Build history of the part. All positions in model axes, mm. Face numbers are marked on the shaded views. A direction names the side the tool comes from. Round coordinates to 2 decimals unless told otherwise and drop trailing zeros. Order: outer loops, then holes, each group sorted by start corner. A loop starts at its lowest first (then second) coordinate and runs counter-clockwise, first axis right, second up. Notation, with made-up numbers: (78.25, 48) -> (110.25, 48) arc R23 ccw to (110.25, 83) -> close; hole circle Ø8 at (-17, -25). An arc over 180 degrees is marked (long way). Write item = value, one per line.
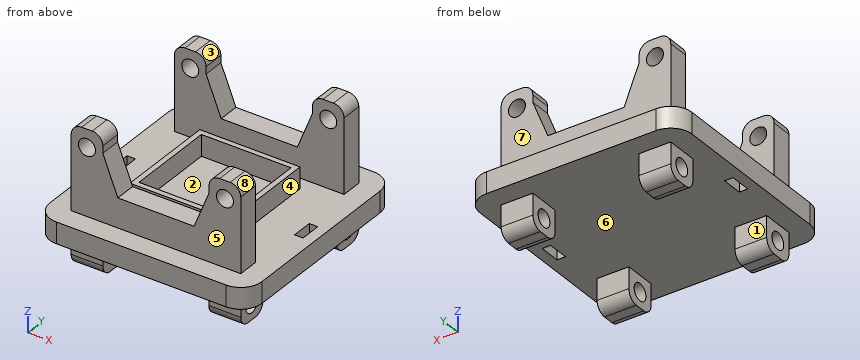
from build123d import *

# Parameters (mm, degrees)
SCHIZZO1_W                   = 100
SCHIZZO1_H                   = 100
ESTRUSIONE_ESTRUSIONE1_DEPTH = 10
RACCORDO1_R                  = 10
SCHIZZO6_W                   = 15
SCHIZZO6_H                   = 15
ESTRUSIONE_ESTRUSIONE2_DEPTH = 15
RACCORDO2_R                  = 5
SCHIZZO7_R                   = 4
TAGLIO_ESTRUSIONE1_DEPTH     = 15
RACCORDO3_R                  = 5
SPECCHIA6_COPY_1_SKETCH_W    = 15
SPECCHIA6_COPY_1_SKETCH_H    = 15
SPECCHIA6_COPY_1_DEPTH       = 15
SPECCHIA6_COPY_2_SKETCH_R    = 4
SPECCHIA6_COPY_2_DEPTH       = 15
RACCORDO3_OF_SPECCHIA6_R     = 5
RACCORDO4_R                  = 5
SCHIZZO8_W                   = 47.3
SCHIZZO8_H                   = 47.3
SCHIZZO8_W_2                 = 42.3
SCHIZZO8_H_2                 = 42.3
ESTRUSIONE_ESTRUSIONE4_DEPTH = 10
SCHIZZO10_W                  = 80
SCHIZZO10_H                  = 10
ESTRUSIONE_ESTRUSIONE6_DEPTH = 40
SCHIZZO11_R                  = 4
TAGLIO_ESTRUSIONE4_DEPTH     = 30
SCHIZZO11_4_R                = 4
TAGLIO_ESTRUSIONE5_DEPTH     = 30
RACCORDO5_R                  = 5
RACCORDO6_R                  = 5
TAGLIO_ESTRUSIONE6_DEPTH     = 30
RACCORDO7_R                  = 5
RACCORDO8_R                  = 5
RACCORDO9_R                  = 5
SCHIZZO15_R                  = 4
TAGLIO_ESTRUSIONE7_DEPTH     = 30
SCHIZZO15_3_R                = 4
TAGLIO_ESTRUSIONE8_DEPTH     = 30
SCHIZZO16_W                  = 4
SCHIZZO16_H                  = 10
TAGLIO_ESTRUSIONE11_DEPTH    = 10


with BuildPart() as part:
    # Schizzo1 → Estrusione-Estrusione1 (new body)
    with BuildSketch(Plane.XY):
        Rectangle(SCHIZZO1_W, SCHIZZO1_H)
    extrude(amount=ESTRUSIONE_ESTRUSIONE1_DEPTH)

    # Raccordo1
    raccordo1_edges = [part.edges().sort_by_distance(p)[0] for p in [
        (50, -50, 5),
        (-50, -50, 5),
        (-50, 50, 5),
        (50, 50, 5),
    ]]
    fillet(raccordo1_edges, radius=RACCORDO1_R)

    # Schizzo6 → Estrusione-Estrusione2 (add)
    with BuildSketch(Plane(origin=(0, 0, 0), x_dir=(-1, 0, 0), z_dir=(0, 0, -1))):
        with Locations((-32.5, 32.5)):
            Rectangle(SCHIZZO6_W, SCHIZZO6_H)
    estrusione_estrusione2 = extrude(amount=ESTRUSIONE_ESTRUSIONE2_DEPTH)

    # Raccordo2
    raccordo2_edges = [part.edges().sort_by_distance(p)[0] for p in [
        (32.5, 25, -15),
        (32.5, 40, -15),
    ]]
    fillet(raccordo2_edges, radius=RACCORDO2_R)

    # Schizzo7 → Taglio-Estrusione1 (cut)
    with BuildSketch(Plane(origin=(40, 0, 0), x_dir=(0, 0, -1), z_dir=(1, 0, 0))):
        with Locations((7.72654806, 32.54210957)):
            Circle(SCHIZZO7_R)
    taglio_estrusione1 = extrude(amount=-TAGLIO_ESTRUSIONE1_DEPTH, mode=Mode.SUBTRACT)

    # Specchia3: Estrusione-Estrusione2, Taglio-Estrusione1 across plane
    add(estrusione_estrusione2.mirror(Plane(origin=(0, 0, 0), x_dir=(0, 0, 1), z_dir=(1, 0, 0))))
    add(taglio_estrusione1.mirror(Plane(origin=(0, 0, 0), x_dir=(0, 0, 1), z_dir=(1, 0, 0))), mode=Mode.SUBTRACT)

    # Raccordo3
    raccordo3_edges = [part.edges().sort_by_distance(p)[0] for p in [
        (-32.5, 40, -15),
        (-32.5, 25, -15),
    ]]
    fillet(raccordo3_edges, radius=RACCORDO3_R)

    # Specchia6: Estrusione-Estrusione2, Taglio-Estrusione1 across plane
    add(estrusione_estrusione2.mirror(Plane.ZX))
    add(taglio_estrusione1.mirror(Plane.ZX), mode=Mode.SUBTRACT)

    # Specchia6 copy 1 sketch → Specchia6 copy 1 (add)
    with BuildSketch(Plane(origin=(0, 0, 0), x_dir=(1, 0, 0), z_dir=(0, 0, -1))):
        with Locations((-32.5, 32.5)):
            Rectangle(SPECCHIA6_COPY_1_SKETCH_W, SPECCHIA6_COPY_1_SKETCH_H)
    extrude(amount=SPECCHIA6_COPY_1_DEPTH)

    # Specchia6 copy 2 sketch → Specchia6 copy 2 (cut)
    with BuildSketch(Plane(origin=(-40, 0, 0), x_dir=(0, 0, -1), z_dir=(-1, 0, 0))):
        with Locations((7.72654806, 32.54210957)):
            Circle(SPECCHIA6_COPY_2_SKETCH_R)
    extrude(amount=-SPECCHIA6_COPY_2_DEPTH, mode=Mode.SUBTRACT)

    # Raccordo3 of Specchia6
    raccordo3_of_specchia6_edges = [part.edges().sort_by_distance(p)[0] for p in [
        (-32.5, -40, -15),
        (-32.5, -25, -15),
    ]]
    fillet(raccordo3_of_specchia6_edges, radius=RACCORDO3_OF_SPECCHIA6_R)

    # Raccordo4
    raccordo4_edges = [part.edges().sort_by_distance(p)[0] for p in [
        (32.5, -40, -15),
        (32.5, -25, -15),
    ]]
    fillet(raccordo4_edges, radius=RACCORDO4_R)

    # Schizzo8 → Estrusione-Estrusione4 (add)
    with BuildSketch(Plane.XY.offset(10)):
        Rectangle(SCHIZZO8_W, SCHIZZO8_H)
        Rectangle(SCHIZZO8_W_2, SCHIZZO8_H_2, mode=Mode.SUBTRACT)
    extrude(amount=ESTRUSIONE_ESTRUSIONE4_DEPTH)

    # Schizzo10 → Estrusione-Estrusione6 (add)
    with BuildSketch(Plane.XY.offset(10)):
        with Locations((0, -35)):
            Rectangle(SCHIZZO10_W, SCHIZZO10_H)
    estrusione_estrusione6 = extrude(amount=ESTRUSIONE_ESTRUSIONE6_DEPTH)

    # Schizzo11 → Taglio-Estrusione4 (cut)
    with BuildSketch(Plane.XZ.offset(40)):
        with Locations((32.539177419, 41.650021723)):
            Circle(SCHIZZO11_R)
    extrude(amount=-TAGLIO_ESTRUSIONE4_DEPTH, mode=Mode.SUBTRACT)

    # Schizzo11_4 → Taglio-Estrusione5 (cut)
    with BuildSketch(Plane.XZ.offset(40)):
        with Locations(Location((-32.539177419, 41.650021723, 0), (0, 0, 270))):
            Circle(SCHIZZO11_4_R)
        with Locations((32.539177419, 41.650021723)):
            Circle(SCHIZZO11_4_R)
    extrude(amount=-TAGLIO_ESTRUSIONE5_DEPTH, mode=Mode.SUBTRACT)

    # Raccordo5
    raccordo5_edges = [part.edges().sort_by_distance(p)[0] for p in [
        (-40, -35, 50),
    ]]
    fillet(raccordo5_edges, radius=RACCORDO5_R)

    # Raccordo6
    raccordo6_edges = [part.edges().sort_by_distance(p)[0] for p in [
        (40, -35, 50),
    ]]
    fillet(raccordo6_edges, radius=RACCORDO6_R)

    # Schizzo14 → Taglio-Estrusione6 (cut)
    with BuildSketch(Plane.XZ.offset(40)):
        Polygon((-25.078354838, 41.650021723), (-25.078354838, 50), (25.078354838, 50), (25.078354838, 41.650021723), (17.979592653, 23.776203366), (-17.979592653, 23.776203366), align=None)
    taglio_estrusione6 = extrude(amount=-TAGLIO_ESTRUSIONE6_DEPTH, mode=Mode.SUBTRACT)

    # Raccordo7
    raccordo7_edges = [part.edges().sort_by_distance(p)[0] for p in [
        (-25.078354838, -35, 50),
    ]]
    fillet(raccordo7_edges, radius=RACCORDO7_R)

    # Raccordo8
    raccordo8_edges = [part.edges().sort_by_distance(p)[0] for p in [
        (25.078354838, -35, 50),
    ]]
    fillet(raccordo8_edges, radius=RACCORDO8_R)

    # Specchia13: Estrusione-Estrusione6 across plane
    add(estrusione_estrusione6.mirror(Plane.ZX))

    # Specchia14: Estrusione-Estrusione6, Taglio-Estrusione6 across plane
    add(estrusione_estrusione6.mirror(Plane.ZX))
    add(taglio_estrusione6.mirror(Plane.ZX), mode=Mode.SUBTRACT)

    # Raccordo9
    raccordo9_edges = [part.edges().sort_by_distance(p)[0] for p in [
        (40, 35, 50),
        (-40, 35, 50),
        (25.078354838, 35, 50),
        (-25.078354838, 35, 50),
    ]]
    fillet(raccordo9_edges, radius=RACCORDO9_R)

    # Schizzo15 → Taglio-Estrusione7 (cut)
    with BuildSketch(Plane(origin=(0, 40, 0), x_dir=(1, 0, 0), z_dir=(0, 1, 0))):
        with Locations(Location((32.539177419, -41.65, 0), (0, 0, 270))):
            Circle(SCHIZZO15_R)
    extrude(amount=-TAGLIO_ESTRUSIONE7_DEPTH, mode=Mode.SUBTRACT)

    # Schizzo15_3 → Taglio-Estrusione8 (cut)
    with BuildSketch(Plane(origin=(0, 40, 0), x_dir=(1, 0, 0), z_dir=(0, 1, 0))):
        with Locations(Location((32.539177419, -41.65, 0), (0, 0, 270))):
            Circle(SCHIZZO15_3_R)
        with Locations((-32.539177419, -41.65)):
            Circle(SCHIZZO15_3_R)
    extrude(amount=-TAGLIO_ESTRUSIONE8_DEPTH, mode=Mode.SUBTRACT)

    # Schizzo16 → Taglio-Estrusione11 (cut)
    with BuildSketch(Plane(origin=(0, 0, 0), x_dir=(-1, 0, 0), z_dir=(0, 0, -1))):
        with Locations((-43, 0)):
            Rectangle(SCHIZZO16_W, SCHIZZO16_H)
        with Locations((43, 0)):
            Rectangle(SCHIZZO16_W, SCHIZZO16_H)
    extrude(amount=-TAGLIO_ESTRUSIONE11_DEPTH, mode=Mode.SUBTRACT)


solid = part.part
Q1. Flat gauge pins, fed straight in: pin 1 (3 mm diameter, centred on x = -8, z = 14.5, fed in from -Y); pin 2 (5 mm diameter, centred on x = 4.5, y = 37, fed in from +Z); pin 3 (7.5 mm diameter, centred on y = 33, z = -6.5, fed in from +X); pin 4 (8 mm diameter, centred on x = 35, z = -3, fed in from -Y). Where does each tip first touch, or does it go through?
Check values:
pin_1 = -40
pin_2 = 23.78
pin_3 = 40
pin_4 = -50
Q2. Cut at C-C, the plane x = -12. List the corners of the cut face in (y, z).
Check values:
outline = (-50, 0) -> (50, 0) -> (50, 10) -> (40, 10) -> (40, 23.78) -> (30, 23.78) -> (30, 10) -> (23.65, 10) -> (23.65, 20) -> (21.15, 20) -> (21.15, 10) -> (-21.15, 10) -> (-21.15, 20) -> (-23.65, 20) -> (-23.65, 10) -> (-30, 10) -> (-30, 23.78) -> (-40, 23.78) -> (-40, 10) -> (-50, 10) -> close
Q3. Probe probe 1 along X at (y, z) = (1, 6); probe 2 along Y at (x, z) = (-16, 17); probe 3 along Y at (x, z) = (32.5, 24.5). List the from-to ranges inside material, lowest first.
Check values:
probe_1 = -50 to -45, -41 to 41, 45 to 50
probe_2 = -40 to -30, -23.65 to -21.15, 21.15 to 23.65, 30 to 40
probe_3 = -40 to -30, 30 to 40
Q4. Cut at A-A, the plane z = 11.5. List the corners of the cut face in (x, y).
Check values:
outline = (-40, -40) -> (40, -40) -> (40, -30) -> (-40, -30) -> close; (-40, 30) -> (40, 30) -> (40, 40) -> (-40, 40) -> close; (-23.65, -23.65) -> (23.65, -23.65) -> (23.65, 23.65) -> (-23.65, 23.65) -> close; hole (-21.15, -21.15) -> (21.15, -21.15) -> (21.15, 21.15) -> (-21.15, 21.15) -> close
Q5. Cut at B-B, the plane y = 27. List the corners of the cut face in (x, z).
Check values:
outline = (-50, 0) -> (-40, 0) -> (-40, -14) -> (-25, -14) -> (-25, 0) -> (25, 0) -> (25, -14) -> (40, -14) -> (40, 0) -> (50, 0) -> (50, 10) -> (-50, 10) -> close
Q6. Cut at D-D, the plane y = 13. List the corners of the cut face in (x, z).
Check values:
outline = (-50, 0) -> (50, 0) -> (50, 10) -> (23.65, 10) -> (23.65, 20) -> (21.15, 20) -> (21.15, 10) -> (-21.15, 10) -> (-21.15, 20) -> (-23.65, 20) -> (-23.65, 10) -> (-50, 10) -> close
Q7. Which spindle directions (+Z, -Z, +X, -X, +Y, -Y) get a long thin tool onto all of the face, cutting with end or side? Do the marked faces 1, 2, 3 and 4. Say none if no direction does.
Check values:
face_1 = -Z, +X, -X
face_2 = +Z
face_3 = +Z, +Y, -Y
face_4 = +Z, +X
Q8. Mould opens along Y. For the marked faces 5, 6, 7 and 8 say: released by +Y, released by -Y, zero draft, split by the parting line, or undercut.
Check values:
face_5 = released by -Y
face_6 = undercut
face_7 = released by +Y
face_8 = zero draft
